```python
from build123d import *

# Parameters (mm, degrees)
F0_R           = 4.6355
F1_DEPTH       = 69.596
F2_D           = 5.588
F2_CBORE_D     = 9.271
F2_CBORE_DEPTH = 7.366
F3_D           = 41.275
F5_D           = 5.1054
F5_DEPTH       = 16.51
F5_TIP         = 1.5338169022


# Not quite as in the source:
# - ends of sketch curves that miss each other by under 0.0002 mm in the source are joined


with BuildPart() as f1:
    # F0 (on Top) → F1 (new body)
    with BuildSketch(Plane.XY):
        with BuildLine():
            Line((0, 20.828), (0, 22.5937319184))
            Line((0, 22.5937319184), (-11.7865243948, 22.593731583))
            ThreePointArc((-11.7865243948, 22.593731583), (-12.6999991591, 18.4785002754), (-13.613476896, 22.593731531))
            Line((-13.613476896, 22.593731531), (-17.0547434947, 26.035))
            Line((-17.0547434947, 26.035), (-23.5585, 26.035))
            Line((-23.5585, 26.035), (-26.035, 23.5585))
            Line((-26.035, 23.5585), (-26.035, 17.0547438789))
            Line((-26.035, 17.0547438789), (-22.5937318573, 13.6134757362))
            ThreePointArc((-22.5937318573, 13.6134757362), (-18.4785, 12.7), (-22.5937318573, 11.7865242638))
            Line((-22.5937318573, 11.7865242638), (-22.5937318573, -11.7865242638))
            ThreePointArc((-22.5937318573, -11.7865242638), (-18.4785, -12.7), (-22.5937318573, -13.6134757362))
            Line((-22.5937318573, -13.6134757362), (-26.035, -17.0547438789))
            Line((-26.035, -17.0547438789), (-26.035, -23.5585))
            Line((-26.035, -23.5585), (-23.5585, -26.035))
            Line((-23.5585, -26.035), (-17.0547438789, -26.035))
            Line((-17.0547438789, -26.035), (-13.6134757362, -22.5937318573))
            ThreePointArc((-13.6134757362, -22.5937318573), (-12.7, -18.4785), (-11.7865242638, -22.5937318573))
            Line((-11.7865242638, -22.5937318573), (11.7865242638, -22.5937318573))
            ThreePointArc((11.7865242638, -22.5937318573), (12.7, -18.4785), (13.6134757362, -22.5937318573))
            Line((13.6134757362, -22.5937318573), (17.0547438789, -26.035))
            Line((17.0547438789, -26.035), (23.5585, -26.035))
            Line((23.5585, -26.035), (26.035, -23.5585))
            Line((26.035, -23.5585), (26.035, -17.0547434947))
            Line((26.035, -17.0547434947), (22.5937319796, -13.6134754743))
            ThreePointArc((22.5937319796, -13.6134754743), (18.4785, -12.7000000097), (22.5937319714, -11.7865245082))
            Line((22.5937319714, -11.7865245082), (22.5937319184, 0))
            Line((22.5937319184, 0), (20.828, 0))
            ThreePointArc((20.828, 0), (-14.7276200386, -14.7276200386), (0, 20.828))
        make_face()
        with Locations((-19.8628, -19.8628)):
            Circle(F0_R, mode=Mode.SUBTRACT)
        with Locations((19.8628, -19.8628)):
            Circle(F0_R, mode=Mode.SUBTRACT)
        with Locations((-19.8628, 19.8628)):
            Circle(F0_R, mode=Mode.SUBTRACT)
        Polygon((0, 22.5937319184), (11.7865243948, 22.5937322538), (8.8899997904, 29.9597321714), (-8.89, 29.9597316654), (-11.7865243948, 22.593731583), align=None)
        with BuildLine():
            Line((26.035, 23.5585), (23.5585, 26.035))
            Line((23.5585, 26.035), (17.0547438789, 26.035))
            Line((17.0547438789, 26.035), (13.6134752367, 22.5937323058))
            ThreePointArc((13.6134752367, 22.5937323058), (12.6999999329, 18.4785002754), (11.7865243948, 22.5937322538))
            Line((11.7865243948, 22.5937322538), (0, 22.5937319184))
            Line((0, 22.5937319184), (0, 20.828))
            ThreePointArc((0, 20.828), (14.7276200386, 14.7276200386), (20.828, 0))
            Line((20.828, 0), (22.5937319184, 0))
            Line((22.5937319184, 0), (22.5937318655, 11.7865242814))
            ThreePointArc((22.5937318655, 11.7865242814), (18.4785, 12.6999999903), (22.5937318573, 13.6134757362))
            Line((22.5937318573, 13.6134757362), (26.035, 17.0547438789))
            Line((26.035, 17.0547438789), (26.035, 23.5585))
        make_face()
        with Locations((19.8628, 19.8628)):
            Circle(F0_R, mode=Mode.SUBTRACT)
        with Locations((19.8628, -19.8628)):
            Circle(F0_R)
        with Locations((19.8628, 19.8628)):
            Circle(F0_R)
        with Locations((-19.8628, 19.8628)):
            Circle(F0_R)
        with Locations((-19.8628, -19.8628)):
            Circle(F0_R)
        with BuildLine():
            ThreePointArc((20.828, 0), (14.7276200386, 14.7276200386), (0, 20.828))
            Line((0, 20.828), (0, 0))
            Line((0, 0), (20.828, 0))
        make_face()
        with BuildLine():
            Line((0, 0), (0, 20.828))
            ThreePointArc((0, 20.828), (-14.7276200386, -14.7276200386), (20.828, 0))
            Line((20.828, 0), (0, 0))
        make_face()
    extrude(amount=-F1_DEPTH)

    # F2 (through all)
    with Locations(Plane.XY):
        with Locations((-19.8628, 19.8628), (19.8628, 19.8628), (19.8628, -19.8628), (-19.8628, -19.8628)):
            CounterBoreHole(F2_D / 2, F2_CBORE_D / 2, F2_CBORE_DEPTH)

    # F3 (through all)
    with Locations(Plane.XY):
        with Locations((0, 0)):
            Hole(F3_D / 2)

    # F5
    with Locations(Plane(origin=(-8.526e-07, 29.9597319184, 0), x_dir=(-1, -2.85e-08, 0), z_dir=(-2.85e-08, 1, 0))):
        with Locations((0, -11.9891270243), (0, -53.7712314358)):
            Hole(F5_D / 2, depth=F5_DEPTH)
            with Locations((0, 0, -(F5_DEPTH + F5_TIP / 2))):  # 118° drill point
                Cone(0, F5_D / 2, F5_TIP, mode=Mode.SUBTRACT)


solid = f1.part
```
Can you work these out from the model? Positions are in its coordinate system, mm. A direction names the side the tool comes from. Coordinates: 2 decimals unless noted, no trailing zeros. Loops run counter-clockwise (first coordinate to the right, second up) from the corner with the lowest first, then second, coordinate; pieces in that order, holes last. Notation, with made-up numbers: (14, 23) - (65, 23) arc R27 ccw to (65, 55) - close; hole circle Ø9 at (-15.75, -4.75). An arc over 180 degrees is marked (long way). Answer as CSV lines item,"result". Start each with the question number.
1) Suppose I cut it at A-A (x = 0). Please give me the cut outline in (y, z).
2) Suppose I cut it at D-D (z = -36.5). Count the separate pieces of the cut face and the enclosed holes in it, plus the area to 3 significant figures.
3) Which directions (+Z, -Z, +X, -X, +Y, -Y) give clear straight access to the entire face, cutting with the end or side of a thin tool? Please do faces 1 (the flat face through (-24.34, 15.36, -34.31)), 2 (the flat face through (-15.36, -24.34, -34.31)), 3 (the flat face through (-19.9, 16.8, -7.366)).
4) Suppose I cut it at B-B (y = -12.7). Please give me the cut outline in (x, z), plus the area to 3 significant figures.
5) Thinking about a two-plate mould opening in Y: for faces 4 (the flat face through (24.779, -24.814, -34.311)), 5 (the flat face through (-20, 26.035, -34)), 6 (the cylindrical face through (-19.499, 22.633, -38.917)), 7 (the cylindrical face through (-0.55, 25.15, -14.48)), which applies, pulls with the +Y half, pulls with the -Y half, needs draft (parallel to the pull), parting line crosses it, or undercut?
6) I need wall thicknesses on line 1 (Y direction, x = -15.5, z = -66); line 2 (X direction, y = -18, z = -36.5) (3 decimals); line 3 (Z direction, x = 19, y = 16). Which ranges of each line are inside material? Lowest first, please. Write a range as from..to.
7) For pin 1 (6 mm diameter, centred on x = 0, z = -11.99, fed in from -Y); pin 2 (4.5 mm diameter, centred on x = 21, y = 19.5, fed in from +Z); pin 3 (6 mm diameter, centred on y = 8, z = -43.5, fed in from +X), each with a flat end and sliding along its axis, tell me the tip position at first contact or that it passes through.
Check result:
1,outline,"(-22.59, -69.6) - (-20.64, -69.6) - (-20.64, 0) - (-22.59, 0) - close; (20.64, -69.6) - (29.96, -69.6) - (29.96, -56.32) - (20.64, -56.32) - close; (20.64, -51.22) - (29.96, -51.22) - (29.96, -14.54) - (20.64, -14.54) - close; (20.64, -9.44) - (29.96, -9.44) - (29.96, 0) - (20.64, 0) - close"
2,separate pieces,"1"
2,enclosed holes,"5"
2,area,"878 mm²"
3,face 1,"+Z, -Z, -X"
3,face 2,"+Z, -Z, -Y"
3,face 3,"+Z"
4,outline,"(-18.48, -69.6) - (-16.27, -69.6) - (-16.27, 0) - (-18.48, 0) - close; (16.27, -69.6) - (18.48, -69.6) - (18.48, 0) - (16.27, 0) - close"
4,area,"308 mm²"
5,face 4,"pulls with the -Y half"
5,face 5,"pulls with the +Y half"
5,face 6,"undercut"
5,face 7,"needs draft"
6,line 1,"y = -24.48..-13.63, 13.63..24.48"
6,line 2,"x = -26.035..-21.945, -17.78..-10.095, 10.095..17.78, 21.945..26.035"
6,line 3,"z = -69.6..-7.37"
7,pin 1,"stops at y = -22.59"
7,pin 2,"stops at z = -7.37"
7,pin 3,"stops at x = 22.59"
